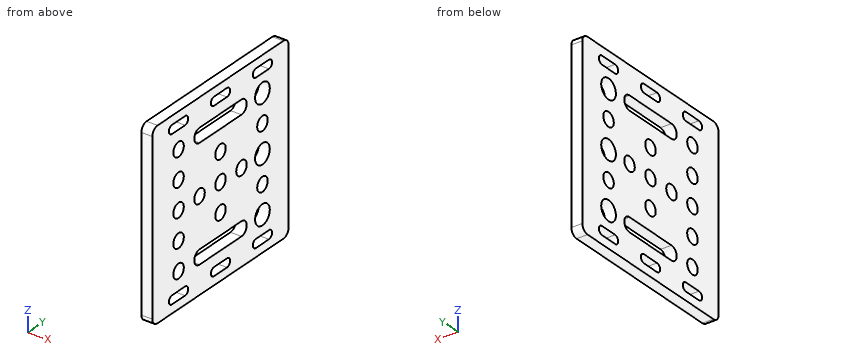
from build123d import *

# Parameters (mm, degrees)
SKETCH1_R           = 2.5
SKETCH1_R_2         = 3.5
BOSS_EXTRUDE1_DEPTH = 3.9


with BuildPart() as part:
    # Sketch1 → Boss-Extrude1 (new body)
    with BuildSketch(Plane(origin=(0, 0, 0), x_dir=(0, 0, -1), z_dir=(1, 0, 0))):
        with BuildLine():
            Line((30, 32.5), (-30, 32.5))
            ThreePointArc((-30, 32.5), (-31.767766953, 31.767766953), (-32.5, 30))
            Line((-32.5, 30), (-32.5, -30))
            ThreePointArc((-32.5, -30), (-31.767766953, -31.767766953), (-30, -32.5))
            Line((-30, -32.5), (30, -32.5))
            ThreePointArc((30, -32.5), (31.767766953, -31.767766953), (32.5, -30))
            Line((32.5, -30), (32.5, 30))
            ThreePointArc((32.5, 30), (31.767766953, 31.767766953), (30, 32.5))
        make_face()
        with Locations((0, -20)):
            Circle(SKETCH1_R, mode=Mode.SUBTRACT)
        with Locations((10, -20)):
            Circle(SKETCH1_R, mode=Mode.SUBTRACT)
        with Locations((-10, -20)):
            Circle(SKETCH1_R, mode=Mode.SUBTRACT)
        with Locations((10, 0)):
            Circle(SKETCH1_R, mode=Mode.SUBTRACT)
        with Locations((0, -10)):
            Circle(SKETCH1_R, mode=Mode.SUBTRACT)
        with Locations((-10, 0)):
            Circle(SKETCH1_R, mode=Mode.SUBTRACT)
        Circle(SKETCH1_R, mode=Mode.SUBTRACT)
        with Locations((0, 10)):
            Circle(SKETCH1_R, mode=Mode.SUBTRACT)
        with Locations((20, -20)):
            Circle(SKETCH1_R, mode=Mode.SUBTRACT)
        with Locations((-20, -20)):
            Circle(SKETCH1_R, mode=Mode.SUBTRACT)
        with Locations((10, 20)):
            Circle(SKETCH1_R, mode=Mode.SUBTRACT)
        with Locations((0, 20)):
            Circle(SKETCH1_R_2, mode=Mode.SUBTRACT)
        with Locations((-10, 20)):
            Circle(SKETCH1_R, mode=Mode.SUBTRACT)
        with Locations((20, 20)):
            Circle(SKETCH1_R_2, mode=Mode.SUBTRACT)
        with Locations((-20, 20)):
            Circle(SKETCH1_R_2, mode=Mode.SUBTRACT)
        with BuildLine():
            Line((26.5, 16.9), (26.5, 23.1))
            ThreePointArc((26.5, 23.1), (28, 24.6), (29.5, 23.1))
            Line((29.5, 23.1), (29.5, 16.9))
            ThreePointArc((29.5, 16.9), (28, 15.4), (26.5, 16.9))
        make_face(mode=Mode.SUBTRACT)
        with BuildLine():
            Line((26.5, -3.1), (26.5, 3.1))
            ThreePointArc((26.5, 3.1), (28, 4.6), (29.5, 3.1))
            Line((29.5, 3.1), (29.5, -3.1))
            ThreePointArc((29.5, -3.1), (28, -4.6), (26.5, -3.1))
        make_face(mode=Mode.SUBTRACT)
        with BuildLine():
            Line((26.5, -23.1), (26.5, -16.9))
            ThreePointArc((26.5, -16.9), (28, -15.4), (29.5, -16.9))
            Line((29.5, -16.9), (29.5, -23.1))
            ThreePointArc((29.5, -23.1), (28, -24.6), (26.5, -23.1))
        make_face(mode=Mode.SUBTRACT)
        with BuildLine():
            Line((-29.5, -23.1), (-29.5, -16.9))
            ThreePointArc((-29.5, -16.9), (-28, -15.4), (-26.5, -16.9))
            Line((-26.5, -16.9), (-26.5, -23.1))
            ThreePointArc((-26.5, -23.1), (-28, -24.6), (-29.5, -23.1))
        make_face(mode=Mode.SUBTRACT)
        with BuildLine():
            Line((17.5, -10), (17.5, 10))
            ThreePointArc((17.5, 10), (20, 12.5), (22.5, 10))
            Line((22.5, 10), (22.5, -10))
            ThreePointArc((22.5, -10), (20, -12.5), (17.5, -10))
        make_face(mode=Mode.SUBTRACT)
        with BuildLine():
            Line((-22.5, -10), (-22.5, 10))
            ThreePointArc((-22.5, 10), (-20, 12.5), (-17.5, 10))
            Line((-17.5, 10), (-17.5, -10))
            ThreePointArc((-17.5, -10), (-20, -12.5), (-22.5, -10))
        make_face(mode=Mode.SUBTRACT)
        with BuildLine():
            Line((-29.5, 16.9), (-29.5, 23.1))
            ThreePointArc((-29.5, 23.1), (-28, 24.6), (-26.5, 23.1))
            Line((-26.5, 23.1), (-26.5, 16.9))
            ThreePointArc((-26.5, 16.9), (-28, 15.4), (-29.5, 16.9))
        make_face(mode=Mode.SUBTRACT)
        with BuildLine():
            Line((-29.5, -3.1), (-29.5, 3.1))
            ThreePointArc((-29.5, 3.1), (-28, 4.6), (-26.5, 3.1))
            Line((-26.5, 3.1), (-26.5, -3.1))
            ThreePointArc((-26.5, -3.1), (-28, -4.6), (-29.5, -3.1))
        make_face(mode=Mode.SUBTRACT)
    extrude(amount=-BOSS_EXTRUDE1_DEPTH)


solid = part.part
Geometry: final body of the model. Coordinates: model frame, mm. Give positions to 0.01 mm unless a question says otherwise; leave off trailing zeros. Loops run counter-clockwise (first coordinate to the right, second up) from the corner with the lowest first, then second, coordinate; pieces in that order, holes last. Notation, with made-up numbers: M 64,-19.5 L 83,-19.5 A25 cw 83,-7.5 Z; hole C -20,76.25 d5. An arc over 180 degrees is marked long. Put each result on its own line as item: value.
1) Cut plane C-C, the plane z = 1.5. Return the cut outline in (x, y), plus the area to 3 significant figures.
Computed values:
outline: M -3.9,-32.5 L 0,-32.5 L 0,-22 L -3.9,-22 Z; M -3.9,-18 L 0,-18 L 0,-12 L -3.9,-12 Z; M -3.9,-8 L 0,-8 L 0,-2 L -3.9,-2 Z; M -3.9,2 L 0,2 L 0,8 L -3.9,8 Z; M -3.9,12 L 0,12 L 0,16.84 L -3.9,16.84 Z; M -3.9,23.16 L 0,23.16 L 0,32.5 L -3.9,32.5 Z
area: 166 mm^2
2) First-contact query: P1, Ø5.5, axis at y = 20, z = 20, coming from the -X side. Flat tip, straight axial feed; report the tip coordinate or a pass-through.
Computed values:
P1: passes through
3) Cut plane D-D, the plane y = 9. Return the cut outline in (x, z).
Computed values:
outline: M -3.9,-32.5 L 0,-32.5 L 0,-22.5 L -3.9,-22.5 Z; M -3.9,-17.5 L 0,-17.5 L 0,-2.29 L -3.9,-2.29 Z; M -3.9,2.29 L 0,2.29 L 0,17.5 L -3.9,17.5 Z; M -3.9,22.5 L 0,22.5 L 0,32.5 L -3.9,32.5 Z
4) Cut plane B-B, the plane y = 0. Give the number of separate pieces and of enclosed holes in the cut face, plus the area to 3 significant figures.
Computed values:
separate pieces: 8
enclosed holes: 0
area: 133 mm^2
5) Material intervals for L1, parallel to Z at x = -0.85, y = 7; L2, parallel to Y at x = -3, z = 0; L3, parallel to Y at x = -2.7, z = -9, sorted ascending. Write a range as from..to.
Computed values:
L1: z = -32.5..-22.5, -17.5..17.5, 22.5..32.5
L2: y = -32.5..-22.5, -17.5..-12.5, -7.5..-2.5, 2.5..7.5, 12.5..16.5, 23.5..32.5
L3: y = -32.5..-22.29, -17.71..-2.29, 2.29..17.71, 22.29..32.5
6) Cut plane A-A, the plane z = 28. Return the cut outline in (x, y), plus the area to 3 significant figures.
Computed values:
outline: M -3.9,-32.5 L 0,-32.5 L 0,-24.6 L -3.9,-24.6 Z; M -3.9,-15.4 L 0,-15.4 L 0,-4.6 L -3.9,-4.6 Z; M -3.9,4.6 L 0,4.6 L 0,15.4 L -3.9,15.4 Z; M -3.9,24.6 L 0,24.6 L 0,32.5 L -3.9,32.5 Z
area: 146 mm^2
